Job drawing, mm, ordinate dimensions from the low corner. One solid piece. Round coordinates to 2 decimals unless told otherwise and drop trailing zeros. Order: outer loops, then holes, each group sorted by start corner. A loop starts at its lowest first (then second) coordinate and runs counter-clockwise, first axis right, second up. Notation, with made-up numbers: (-33.5, 24) -> (25.5, 24) arc R22 cw to (25.5, 35) -> close; hole circle Ø11 at (53, 78.25). An arc over 180 degrees is marked (long way). Answer as a JSON object with one key per item and string values. Group by question number.
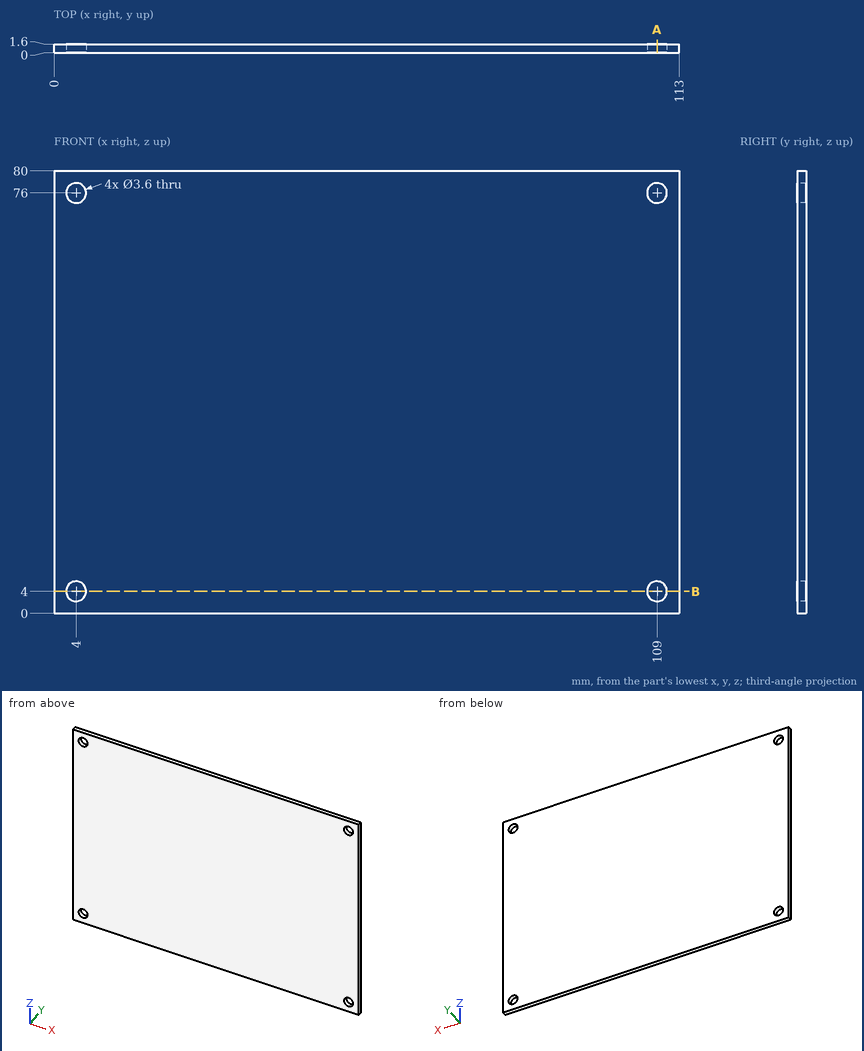
Q1. Band-saw the part on A-A (x = 109). List the corners of the cut face in (y, z), plus the area to 3 significant figures.
Q2. Band-saw the part on B-B (z = 4). List the corners of the cut face in (x, y), plus the area to 3 significant figures.
Q3. Wall check: line 1 (X direction, y = 0.4, z = 76); line 2 (Z direction, x = 109, y = 1.1); line 3 (X direction, y = 0.65, z = 74.5). Give the ranges that are in metal, low to high. Write a range as [from, to].
Q4. Drop a flat-ended pin along its axis: pin 1 Ø3 at (x, z) = (109, 4) entering from -Y. Give the stop position or say it passes through.
Completed:
{
 "1": {"outline": "(0, 0) -> (1.6, 0) -> (1.6, 2.2) -> (0, 2.2) -> close; (0, 5.8) -> (1.6, 5.8) -> (1.6, 74.2) -> (0, 74.2) -> close; (0, 77.8) -> (1.6, 77.8) -> (1.6, 80) -> (0, 80) -> close", "area": "116 mm2"},
 "2": {"outline": "(0, 0) -> (2.2, 0) -> (2.2, 1.6) -> (0, 1.6) -> close; (5.8, 0) -> (107.2, 0) -> (107.2, 1.6) -> (5.8, 1.6) -> close; (110.8, 0) -> (113, 0) -> (113, 1.6) -> (110.8, 1.6) -> close", "area": "169 mm2"},
 "3": {"line 1": "[0, 2.2], [5.8, 107.2], [110.8, 113]", "line 2": "[0, 2.2], [5.8, 74.2], [77.8, 80]", "line 3": "[0, 3.01], [4.99, 108.01], [109.99, 113]"},
 "4": {"pin 1": "through"}
}
